```python
from build123d import *

# Parameters (mm, degrees)
SKETCH_1_W          = 40
SKETCH_1_H          = 48
SKETCH_1_R          = 1.75
EXTRUDE_1_DEPTH     = 4
SKETCH_2_W          = 40
SKETCH_2_H          = 7.75
EXTRUDE_5_DEPTH     = 20.5
SKETCH_4_W          = 40
SKETCH_4_H          = 36
EXTRUDE_6_DEPTH     = 3
FILLET_4_R          = 5
FILLET_11_R         = 5
SKETCH_8_W          = 40
SKETCH_8_H          = 48
EXTRUDE_8_DEPTH     = 4
SKETCH_9_W          = 40
SKETCH_9_H          = 60
EXTRUDE_9_DEPTH     = 4
SKETCH_10_R         = 1.6
CUT_EXTRUDE_1_DEPTH = 46.345892868
SKETCH_12_W         = 40
SKETCH_12_H         = 48
EXTRUDE_11_DEPTH    = 2
SKETCH_13_R         = 2.15
CUT_EXTRUDE_2_DEPTH = 50.216359069


with BuildPart() as part:
    # 草图1 → 凸台-拉伸1 (new body)
    with BuildSketch(Plane(origin=(0, 0, 0), x_dir=(1, 0, 0), z_dir=(0, 1, 0))):
        Rectangle(SKETCH_1_W, SKETCH_1_H)
        with Locations(Location((11.45, 14, 0), (0, 0, 270))):
            Circle(SKETCH_1_R, mode=Mode.SUBTRACT)
        with Locations(Location((-11.45, 14, 0), (0, 0, 270))):
            Circle(SKETCH_1_R, mode=Mode.SUBTRACT)
        with Locations(Location((-11.45, -14, 0), (0, 0, 270))):
            Circle(SKETCH_1_R, mode=Mode.SUBTRACT)
        with Locations(Location((11.45, -14, 0), (0, 0, 270))):
            Circle(SKETCH_1_R, mode=Mode.SUBTRACT)
        with BuildLine():
            Line((-2.45, -15.5), (-2.45, 15.5))
            ThreePointArc((-2.45, 15.5), (0, 17.95), (2.45, 15.5))
            Line((2.45, 15.5), (2.45, -15.5))
            ThreePointArc((2.45, -15.5), (0, -17.95), (-2.45, -15.5))
        make_face(mode=Mode.SUBTRACT)
    extrude(amount=EXTRUDE_1_DEPTH)

    # 草图2 → 凸台-拉伸5 (add)
    with BuildSketch(Plane(origin=(0, 4, 0), x_dir=(1, 0, 0), z_dir=(0, 1, 0))):
        with Locations((0, -14.125)):
            Rectangle(SKETCH_2_W, SKETCH_2_H)
        with Locations((0, 14.125)):
            Rectangle(SKETCH_2_W, SKETCH_2_H)
    extrude(amount=EXTRUDE_5_DEPTH)

    # 草图4 → 凸台-拉伸6 (add)
    with BuildSketch(Plane(origin=(0, 24.5, 0), x_dir=(1, 0, 0), z_dir=(0, 1, 0))):
        Rectangle(SKETCH_4_W, SKETCH_4_H)
    extrude(amount=EXTRUDE_6_DEPTH)

    # 圆角4
    fillet_4_edges = [part.edges().sort_by_distance(p)[0] for p in [
        (0, 4, -18),
    ]]
    fillet(fillet_4_edges, radius=FILLET_4_R)

    # 圆角11
    fillet_11_edges = [part.edges().sort_by_distance(p)[0] for p in [
        (0, 4, 18),
    ]]
    fillet(fillet_11_edges, radius=FILLET_11_R)

    # 草图8 → 凸台-拉伸8 (add)
    with BuildSketch(Plane(origin=(0, 27.5, 0), x_dir=(1, 0, 0), z_dir=(0, 1, 0))):
        Rectangle(SKETCH_8_W, SKETCH_8_H)
    extrude(amount=EXTRUDE_8_DEPTH)

    # 草图9 → 凸台-拉伸9 (add)
    with BuildSketch(Plane.XZ):
        Rectangle(SKETCH_9_W, SKETCH_9_H)
    extrude(amount=-EXTRUDE_9_DEPTH)

    # 草图10 → 切除-拉伸1 (cut, through all)
    with BuildSketch(Plane(origin=(0, 4, 0), x_dir=(1, 0, 0), z_dir=(0, 1, 0))):
        with Locations(Location((17, 27, 0), (0, 0, 270))):
            Circle(SKETCH_10_R)
        with Locations(Location((-17, -27, 0), (0, 0, 270))):
            Circle(SKETCH_10_R)
        with Locations(Location((17, -27, 0), (0, 0, 270))):
            Circle(SKETCH_10_R)
        with Locations(Location((-17, 27, 0), (0, 0, 270))):
            Circle(SKETCH_10_R)
    extrude(amount=-CUT_EXTRUDE_1_DEPTH, mode=Mode.SUBTRACT)

    # 草图12 → 凸台-拉伸11 (add)
    with BuildSketch(Plane(origin=(0, 31.5, 0), x_dir=(1, 0, 0), z_dir=(0, 1, 0))):
        Rectangle(SKETCH_12_W, SKETCH_12_H)
    extrude(amount=EXTRUDE_11_DEPTH)

    # 草图13 → 切除-拉伸2 (cut, through all)
    with BuildSketch(Plane(origin=(0, 33.5, 0), x_dir=(1, 0, 0), z_dir=(0, 1, 0))):
        with Locations(Location((-10, 0, 0), (0, 0, 270))):
            Circle(SKETCH_13_R)
        with Locations(Location((0, 0, 0), (0, 0, 270))):
            Circle(SKETCH_13_R)
    extrude(amount=-CUT_EXTRUDE_2_DEPTH, mode=Mode.SUBTRACT)


solid = part.part
```
The model under review builds one solid part; all positions refer to its coordinate system, in mm. A direction names the side the tool comes from. Give positions to 0.01 mm unless a question says otherwise; leave off trailing zeros. Write each loop counter-clockwise with the first axis right and the second up, starting at its lowest first coordinate (ties: lowest second). Pieces come first, ordered by that corner, then holes. Notation, with made-up numbers: (6.5, 44) - (62.5, 44) arc R10 cw to (62.5, 52) - close; hole circle Ø4 at (50.25, -7). An arc over 180 degrees is marked (long way). Answer in a Markdown table with one row per item. Add a question column.
1. Wall thickness on line 1 along X through (y, z) = (2, 0); line 2 along Z through (x, y) = (-5.5, 22); line 3 along Y through (x, z) = (15, -9): over which ranges is each line inside the solid? List them lowest first. Write a range as [from, to].
2. Draft analysis for pull direction X (two halves, no side actions). For faces 1 (the cylindrical face through (-7.87, 29.06, -0.28)), 2 (the flat face through (-20, 28, 0)), 3 (the flat face through (0, 4, -26)), state which applies: +X half, -X half, draft (parallel to the pull), parting line (faces both ways), or undercut.
3. We need section B-B on y = 11. Write out the cut boundary in (x, z).
4. We need section D-D on z = -27. Write out the cut boundary in (x, y).
5. We need section A-A on x = -17. Write out the cut boundary in (y, z).
6. We need section C-C on z = 7.5. Write out the cut boundary in (x, y), then the cut area to 3 significant figures.
7. Tool access review of faces 4 (the flat face through (0, 30, -24)), 5 (the cylindrical face through (0, 6, 19)), 6 (the cylindrical face through (0, 5, -20)), 7 (the flat face through (-0.3, 24.5, -2.4)), 8 (the cylindrical face through (-1.308, 2.028, -1.706)): name each direction out of +Z, -Z, +X, -X, +Y, -Y from which nothing blocks a thin tool from reaching the whole face with its end or side.
8. Insertion check: P1, Ø3.5, axis at x = 17, z = -27, coming from the +Y side; P2, Ø6, axis at x = -3.5, y = 10, coming from the +Z side; P3, Ø6.5, axis at x = -5, y = 31.5, coming from the +Z side. Each pin has a flat end and moves straight along its axis. Give the tip position at first contact, or say it passes through.
Ans:
| question | item | result |
|---|---|---|
| 1 | line 1 | x = [-20, -12.15], [-7.85, -2.15], [2.15, 20] |
| 1 | line 2 | z = [-18, -10.25], [10.25, 18] |
| 1 | line 3 | y = [0, 4], [24.5, 33.5] |
| 2 | face 1 | undercut |
| 2 | face 2 | -X half |
| 2 | face 3 | draft |
| 3 | outline | (-20, -18) - (20, -18) - (20, -10.25) - (-20, -10.25) - close; (-20, 10.25) - (20, 10.25) - (20, 18) - (-20, 18) - close |
| 4 | outline | (-20, 0) - (-18.6, 0) - (-18.6, 4) - (-20, 4) - close; (-15.4, 0) - (15.4, 0) - (15.4, 4) - (-15.4, 4) - close; (18.6, 0) - (20, 0) - (20, 4) - (18.6, 4) - close |
| 5 | outline | (0, -30) - (4, -30) - (4, -28.6) - (0, -28.6) - close; (0, -25.4) - (4, -25.4) - (4, -23) arc R5 cw to (9, -18) - (27.5, -18) - (27.5, -24) - (33.5, -24) - (33.5, 24) - (27.5, 24) - (27.5, 18) - (9, 18) arc R5 cw to (4, 23) - (4, 25.4) - (0, 25.4) - close; (0, 28.6) - (4, 28.6) - (4, 30) - (0, 30) - close; hole (4, -10.25) - (24.5, -10.25) - (24.5, 10.25) - (4, 10.25) - close |
| 6 | outline | (-20, 0) - (20, 0) - (20, 4) - (-20, 4) - close; (-20, 24.5) - (20, 24.5) - (20, 33.5) - (-20, 33.5) - close |
| 6 | area | 520 mm^2 |
| 7 | face 4 | -Z, +X, -X, +Y |
| 7 | face 5 | +Z, +X, -X |
| 7 | face 6 | -Z, +X, -X |
| 7 | face 7 | +X, -X |
| 7 | face 8 | +Y, -Y |
| 8 | P1 | stops at y = 4 |
| 8 | P2 | stops at z = 18.42 |
| 8 | P3 | stops at z = 24 |
